```python
from build123d import *

# Parameters (mm, degrees)
SKETCH1_W           = 60
SKETCH1_H           = 51
BOSS_EXTRUDE1_DEPTH = 20
SKETCH2_W           = 15
SKETCH2_H           = 41
CUT_EXTRUDE1_DEPTH  = 20
SKETCH3_R           = 10
CUT_EXTRUDE2_DEPTH  = 20
SKETCH4_R           = 3.3
CUT_EXTRUDE3_DEPTH  = 20
SKETCH7_W           = 1.141811335
SKETCH7_H           = 10.046427162
CUT_EXTRUDE4_DEPTH  = 20
SCALE1_SCALE        = 0.8
SCALE2_SCALE        = 0.5


with BuildPart() as part:
    # Sketch1 → Boss-Extrude1 (new body)
    with BuildSketch(Plane.XY):
        with Locations((-612.687747036, 357.503952569)):
            Rectangle(SKETCH1_W, SKETCH1_H)
    extrude(amount=BOSS_EXTRUDE1_DEPTH)

    # Sketch2 → Cut-Extrude1 (cut)
    with BuildSketch(Plane.XY.offset(20)):
        with Locations((-635.187747036, 362.503952569)):
            Rectangle(SKETCH2_W, SKETCH2_H)
        with Locations((-590.187747036, 362.503952569)):
            Rectangle(SKETCH2_W, SKETCH2_H)
    extrude(amount=-CUT_EXTRUDE1_DEPTH, mode=Mode.SUBTRACT)

    # Sketch3 → Cut-Extrude2 (cut)
    with BuildSketch(Plane.XY.offset(20)):
        with Locations((-613.095017258, 363.003952569)):
            Circle(SKETCH3_R)
    extrude(amount=-CUT_EXTRUDE2_DEPTH, mode=Mode.SUBTRACT)

    # Sketch4 → Cut-Extrude3 (cut)
    with BuildSketch(Plane(origin=(0, 342.003952569, 0), x_dir=(1, 0, 0), z_dir=(0, 1, 0))):
        with Locations(Location((-635.187747036, -10, 0), (0, 0, 270))):
            Circle(SKETCH4_R)
        with Locations(Location((-590.187747036, -10, 0), (0, 0, 270))):
            Circle(SKETCH4_R)
    extrude(amount=-CUT_EXTRUDE3_DEPTH, mode=Mode.SUBTRACT)

    # Sketch7 → Cut-Extrude4 (cut)
    with BuildSketch(Plane.XY.offset(20)):
        with Locations((-612.703432528, 377.980738988)):
            Rectangle(SKETCH7_W, SKETCH7_H)
    extrude(amount=-CUT_EXTRUDE4_DEPTH, mode=Mode.SUBTRACT)


with BuildPart() as part_1:
    # Scale1: scaled about (-612.600600691, 352.463239706, 10)
    add(part.part.scale(SCALE1_SCALE).moved(Location((-122.520120138, 70.492647941, 2))))


with BuildPart() as part_2:
    # Scale2: scaled about (-612.600600691, 352.463239706, 10)
    add(part_1.part.scale(SCALE2_SCALE).moved(Location((-306.300300345, 176.231619853, 5))))


solid = part_2.part
```
Could you check a few things on this model? Use its own coordinates, in mm. A direction names the side the tool comes from. Coordinates: 2 decimals unless noted, no trailing zeros. Loops run counter-clockwise (first coordinate to the right, second up) from the corner with the lowest first, then second, coordinate; pieces in that order, holes last.
1) Which directions (+Z, -Z, +X, -X, +Y, -Y) give clear straight access to the entire face, cutting with the end or side of a thin tool? Please do faces 5 (the face through (-612.87, 363, 10)), 6 (the face through (-623, 348.28, 11)), 7 (the face through (-605, 348.28, 11)), 8 (the face through (-616, 364.68, 10)).
Reported:
face 5: +Z, -Z, +Y
face 6: +Z, -Z, -X, +Y
face 7: +Z, -Z, +X, +Y
face 8: +Z, -Z, +X, -X, +Y
2) Please list where these lines run through material, in increasing order: line 1 along X through (y, z) = (346.1, 10); line 2 along X through (y, z) = (363.5, 10.25); line 3 along Y through (x, z) = (-620.75, 6.5).
Reported:
line 1: x = -624.64 to -622.96, -620.32 to -604.96, -602.32 to -600.64
line 2: x = -618.64 to -612.87, -612.41 to -606.64
line 3: y = 344.28 to 348.28
3) Thinking about a two-plate mould opening in Z: for faces 1 (the face through (-613, 352, 14)), 2 (the face through (-622.924, 346.308, 9.714)), 3 (the face through (-606.635, 356, 10)), 4 (the face through (-604.924, 346.308, 9.714)), which applies, released by +Z, released by -Z, zero draft, split by the parting line, or undercut?
Reported:
face 1: released by +Z
face 2: undercut
face 3: zero draft
face 4: undercut
4) Imagine slicing it at A-A (y = 363). List the corners of the cut face in (x, z) for me, and give its area (3 significant figures).
Reported:
outline: (-618.64, 6) - (-612.87, 6) - (-612.87, 14) - (-618.64, 14) - close; (-612.41, 6) - (-606.64, 6) - (-606.64, 14) - (-612.41, 14) - close
area: 92.3 mm2
5) Will these pins go through, and if not, where does the flat tip stop? pin 1 Ø4 at (y, z) = (351.5, 9) entering from -X; pin 2 Ø4.5 at (y, z) = (362.5, 11.5) entering from +X; pin 3 Ø1.8 at (x, z) = (-622, 11.5) entering from +Y; pin 4 Ø12 at (x, y) = (-605.5, 354) entering from -Z.
Reported:
pin 1: stops at x = -618.64
pin 2: stops at x = -606.64
pin 3: stops at y = 348.28
pin 4: stops at z = 6
6) Imagine slicing it at C-C (x = -615.75). List the corners of the cut face in (y, z) for me, and give its area (3 significant figures).
Reported:
outline: (344.28, 6) - (353.98, 6) - (353.98, 14) - (344.28, 14) - close; (359.38, 6) - (364.68, 6) - (364.68, 14) - (359.38, 14) - close
area: 120 mm2
7) Imagine slicing it at B-B (z = 10). List the corners of the cut face in (x, y) for me.
Reported:
outline: (-624.64, 344.28) - (-622.96, 344.28) - (-622.96, 348.28) - (-624.64, 348.28) - close; (-620.32, 344.28) - (-604.96, 344.28) - (-604.96, 348.28) - (-606.64, 348.28) - (-606.64, 364.68) - (-612.41, 364.68) - (-612.41, 360.66) arc R4 cw (long way) to (-612.87, 360.68) - (-612.87, 364.68) - (-618.64, 364.68) - (-618.64, 348.28) - (-620.32, 348.28) - close; (-602.32, 344.28) - (-600.64, 344.28) - (-600.64, 348.28) - (-602.32, 348.28) - close
8) Imagine slicing it at D-D (z = 12.25). List the corners of the cut face in (x, y) for me.
Reported:
outline: (-624.64, 344.28) - (-600.64, 344.28) - (-600.64, 348.28) - (-606.64, 348.28) - (-606.64, 364.68) - (-612.41, 364.68) - (-612.41, 360.66) arc R4 cw (long way) to (-612.87, 360.68) - (-612.87, 364.68) - (-618.64, 364.68) - (-618.64, 348.28) - (-624.64, 348.28) - close
